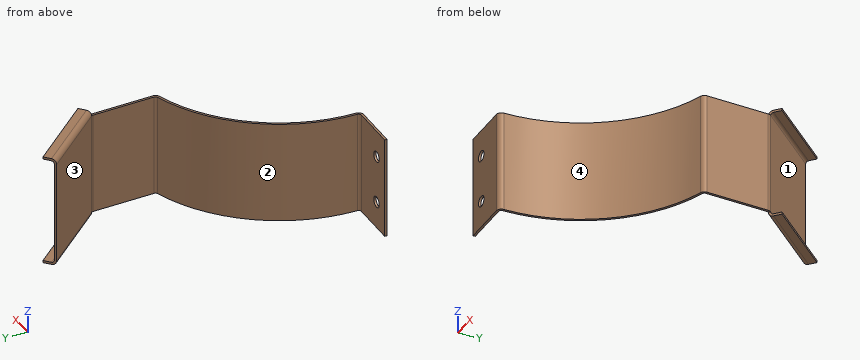
```python
from build123d import *

# Parameters (mm, degrees)
BASE_FLANGE1_DEPTH           = 119.6975
EDGE_FLANGE1_DEPTH           = 119.6975
EDGE_FLANGE2_STRIP_CUT_DEPTH = 119.6975
EDGE_FLANGE2_DEPTH           = 119.6975
EDGE_FLANGE3_DEPTH           = 119.6975
SKETCH20_R                   = 6.35
CUT_EXTRUDE1_DEPTH           = 2.65684
EDGE_FLANGE4_DEPTH           = 100.444394506
EDGE_FLANGE5_DEPTH           = 100.444394506


# Sheet-metal steps are written as plain solids
with BuildPart() as part:
    # Sketch1 → Base-Flange1 (new body)
    with BuildSketch(Plane.XY):
        with BuildLine():
            ThreePointArc((-50.8, 170.388379885), (-140.856418383, 108.500273734), (-177.710803869, 5.63118))
            Line((-177.710803869, 5.63118), (-180.366311024, 5.715325918))
            ThreePointArc((-180.366311024, 5.715325918), (-142.961215721, 110.121577824), (-51.559097143, 172.934469105))
            Line((-51.559097143, 172.934469105), (-50.8, 170.388379885))
        make_face()
    extrude(amount=BASE_FLANGE1_DEPTH)

    # Edge-Flange1 section (across the edge) → Edge-Flange1 (add)
    with BuildSketch(Plane(origin=(-49.291175996, 173.610632552, 119.6975), x_dir=(-0.9999999996342678, -2.7045604981568168e-05, 0), z_dir=(0, 0, -1))):
        with BuildLine():
            Line((-2.65684, 2.366572064), (-2.65684, 76.2))
            Line((-2.65684, 76.2), (0, 76.2))
            Line((0, 76.2), (0, 2.366572064))
            ThreePointArc((0, 2.366572064), (0.62936233, 0.469112223), (2.267939433, -0.676102109))
            Line((2.267939433, -0.676102109), (1.508911151, -3.222211858))
            ThreePointArc((1.508911151, -3.222211858), (-1.500827273, -1.118682173), (-2.65684, 2.366572064))
        make_face()
    extrude(amount=EDGE_FLANGE1_DEPTH)

    # Edge-Flange2 strip (across the edge) → Edge-Flange2 strip cut (cut)
    with BuildSketch(Plane(origin=(-49.293236871, 249.810632524, 119.6975), x_dir=(-0.7660270582590358, -0.6428083275868537, 0), z_dir=(0, 0, -1))):
        Polygon((-12.205285278, 10.412383287), (-1.292448625, -2.593029), (0.742808893, -0.885245167), (-10.17002776, 12.12016712), align=None)
    extrude(amount=EDGE_FLANGE2_STRIP_CUT_DEPTH, mode=Mode.SUBTRACT)

    # Edge-Flange2 section (across the edge) → Edge-Flange2 (add)
    with BuildSketch(Plane(origin=(-49.293236871, 249.810632524, 119.6975), x_dir=(-0.7660270582590358, -0.6428083275868537, 0), z_dir=(0, 0, -1))):
        with BuildLine():
            Line((-2.65684, 1.155605494), (-2.65684, 101.6))
            Line((-2.65684, 101.6), (0, 101.6))
            Line((0, 101.6), (0, 1.155605494))
            ThreePointArc((0, 1.155605494), (0.191475929, 0.069691539), (0.742808893, -0.885245167))
            Line((0.742808893, -0.885245167), (-1.292448625, -2.593029))
            ThreePointArc((-1.292448625, -2.593029), (-2.305137014, -0.839001259), (-2.65684, 1.155605494))
        make_face()
    extrude(amount=EDGE_FLANGE2_DEPTH)

    # Edge-Flange3 section (across the edge) → Edge-Flange3 (add)
    with BuildSketch(Plane(origin=(-180.46686781, 2.541918706, 0), x_dir=(0.0316714285714251, 0.9994983344719717, 0), z_dir=(0, 0, 1))):
        with BuildLine():
            Line((-2.65684, 3.175), (-2.65684, 57.15))
            Line((-2.65684, 57.15), (0, 57.15))
            Line((0, 57.15), (0, 3.175))
            ThreePointArc((0, 3.175), (0.92993597, 0.92993597), (3.175, 0))
            Line((3.175, 0), (3.175, -2.65684))
            ThreePointArc((3.175, -2.65684), (-0.948733611, -0.948733611), (-2.65684, 3.175))
        make_face()
    extrude(amount=EDGE_FLANGE3_DEPTH)

    # Sketch20 → Cut-Extrude1 (cut)
    with BuildSketch(Plane(origin=(-0.100556786, -3.173407212, 0), x_dir=(0.9994983344719716, -0.03167142857142512, 0), z_dir=(0.03167142857142512, 0.9994983344719717, 0))):
        with Locations(Location((-218.55684, -31.75, 0), (0, 0, 180))):
            Circle(SKETCH20_R)
        with Locations(Location((-218.55684, -87.9475, 0), (0, 0, 180))):
            Circle(SKETCH20_R)
    extrude(amount=-CUT_EXTRUDE1_DEPTH, mode=Mode.SUBTRACT)

    # Edge-Flange4 section (across the edge) → Edge-Flange4 (add)
    with BuildSketch(Plane(origin=(-112.567351624, 329.34682052, 122.8725), x_dir=(0, 0, -1), z_dir=(0.6428083275868537, -0.7660270582590358, 0))):
        with BuildLine():
            Line((-2.65684, 3.175), (-2.65684, 12.7))
            Line((-2.65684, 12.7), (0, 12.7))
            Line((0, 12.7), (0, 3.175))
            ThreePointArc((0, 3.175), (0.92993597, 0.92993597), (3.175, 0))
            Line((3.175, 0), (3.175, -2.65684))
            ThreePointArc((3.175, -2.65684), (-0.948733611, -0.948733611), (-2.65684, 3.175))
        make_face()
    extrude(amount=EDGE_FLANGE4_DEPTH)

    # Edge-Flange5 section (across the edge) → Edge-Flange5 (add)
    with BuildSketch(Plane(origin=(-48.000858376, 252.403696478, -3.175), x_dir=(0, 0, 1), z_dir=(-0.642808327586854, 0.7660270582590356, 0))):
        with BuildLine():
            Line((-2.65684, 3.175), (-2.65684, 12.7))
            Line((-2.65684, 12.7), (0, 12.7))
            Line((0, 12.7), (0, 3.175))
            ThreePointArc((0, 3.175), (0.92993597, 0.92993597), (3.175, 0))
            Line((3.175, 0), (3.175, -2.65684))
            ThreePointArc((3.175, -2.65684), (-0.948733611, -0.948733611), (-2.65684, 3.175))
        make_face()
    extrude(amount=EDGE_FLANGE5_DEPTH)


solid = part.part
```
Geometry: final body of the model. Coordinates: model frame, mm. Face numbers are marked on the shaded views. Give positions to 0.01 mm unless a question says otherwise; leave off trailing zeros. Loops run counter-clockwise (first coordinate to the right, second up) from the corner with the lowest first, then second, coordinate; pieces in that order, holes last. Notation, with made-up numbers: (36.25, 47) -> (82.25, 47) arc R17 ccw to (82.25, 60) -> close; hole circle Ø4 at (33.5, 52.25). An arc over 180 degrees is marked (long way). Return JSON: item names as keys, results as strings.
Item 1: Line query: line 1 (X direction, y = 198.5, z = 101) (3 decimals); line 2 (Y direction, x = -109, z = 21); line 3 (Z direction, x = -175.5, y = 33). Output: solid intervals per line, ascending.
Filled in:
{"line 1": "-49.292 to -46.635", "line 2": "140.47 to 143.82, 320.96 to 325.1", "line 3": "0 to 119.7"}
Item 2: Section A-A, the plane z = 11. Output: boundary loops of the cut face in (x, y) (3 decimals), plus the area to 3 significant figures.
Filled in:
{"outline": "(-237.672, 1.696) -> (-183.724, -0.013) arc R5.832 ccw to (-177.711, 5.631) arc R177.8 cw to (-50.8, 170.388) arc R5.832 ccw to (-46.634, 175.977) -> (-46.636, 248.655) arc R5.832 ccw to (-48.001, 252.404) -> (-112.567, 329.347) -> (-114.603, 327.639) -> (-50.036, 250.696) arc R3.175 cw to (-49.293, 248.655) -> (-49.291, 175.977) arc R3.175 cw to (-51.559, 172.934) arc R180.457 ccw to (-180.366, 5.715) arc R3.175 cw to (-183.64, 2.642) -> (-237.588, 4.352) -> close", "area": "1,240 mm^2"}
Item 3: Mould query, pull axis Y, two halves, no side actions, for the marked faces 1, 2, 3 and 4. Classes: released by +Y, released by -Y, zero draft, split by the parting line, or undercut.
Filled in:
{"face 1": "released by +Y", "face 2": "undercut", "face 3": "undercut", "face 4": "released by -Y"}
Item 4: Pin query (flat end, axial travel): P1, Ø1, axis at y = 183.5, z = 46.5, coming from the -X side; P2, Ø8, axis at y = 252, z = 53, coming from the +X side; P3, Ø2, axis at x = -138.5, z = 55.5, coming from the -Y side. Return the tip coordinate at first contact, or that it passes through.
Filled in:
{"P1": "x = -49.29", "P2": "x = -46.64", "P3": "y = 110.24"}
Item 5: Section C-C, the plane x = -148.5. Output: boundary loops of the cut face in (y, z), plus the area to 3 significant figures.
Filled in:
{"outline": "(97.78, 0) -> (102.53, 0) -> (102.53, 119.7) -> (97.78, 119.7) -> close", "area": "569 mm^2"}
